Design review of the part built by this model. Coordinates are the model's own, in mm. A direction names the side the tool comes from. Give positions to 0.01 mm unless a question says otherwise; leave off trailing zeros. Order: outer loops, then holes, each group sorted by start corner. A loop starts at its lowest first (then second) coordinate and runs counter-clockwise, first axis right, second up. Notation, with made-up numbers: (-21.5, -5) -> (26.5, -5) arc R33 cw to (26.5, 33) -> close; hole circle Ø1 at (-14, 10). An arc over 180 degrees is marked (long way). Answer in a Markdown table with one row per item. Add a question column.
```python
from build123d import *

# Parameters (mm, degrees)
F0_W      = 10
F0_H      = 104
F1_DEPTH  = 10
F2_W      = 10
F2_H      = 2
F3_DEPTH  = 15
F4_W      = 10
F4_H      = 2
F5_DEPTH  = 30
F7_DEPTH  = 10.001
F8_R      = 0.99999
F9_W      = 3
F9_H      = 15
F10_DEPTH = 7


# Not quite as in the source:
# - a fillet or chamfer is up to 0.001 mm smaller than in the source, because OpenCascade refuses the exact size


with BuildPart() as f1:
    # F0 (on Top) → F1 (new body)
    with BuildSketch(Plane.XY):
        Rectangle(F0_W, F0_H)
    extrude(amount=F1_DEPTH)

    # F2 (on face) → F3 (join)
    with BuildSketch(Plane.XY.offset(10)):
        with Locations((0, -51)):
            Rectangle(F2_W, F2_H)
    extrude(amount=F3_DEPTH)

    # F4 (on face) → F5 (join)
    with BuildSketch(Plane.XY.offset(10)):
        with Locations((0, 51)):
            Rectangle(F4_W, F4_H)
    extrude(amount=F5_DEPTH)

    # F6 (on face) → F7 (cut, through all)
    with BuildSketch(Plane.YZ.offset(5)):
        Polygon((47, 5), (-30.8395786217, 0), (47, 0), align=None)
    extrude(amount=-F7_DEPTH, mode=Mode.SUBTRACT)

    # F8 (radius 1 in the source; OpenCascade refuses exactly that, so slightly less here)
    f8_edges = [f1.edges().sort_by_distance(p)[0] for p in [
        (0, 50, 40),
        (0, 52, 40),
        (0, -52, 25),
        (0, -50, 25),
        (0, 50, 10),
        (0, -50, 10),
    ]]
    fillet(f8_edges, radius=F8_R)

    # F9 (on face) → F10 (cut)
    with BuildSketch(Plane(origin=(-5, 0, 0), x_dir=(0, -1, 0), z_dir=(-1, 0, 0))):
        with Locations((50.5, 17.5)):
            Rectangle(F9_W, F9_H)
    extrude(amount=-F10_DEPTH, mode=Mode.SUBTRACT)


solid = f1.part
```
1) For L1, parallel to Y at x = 4.5, z = 17.5; L2, parallel to Y at x = -1, z = 32; L3, parallel to Z at x = 3.5, y = -32, list the stretches that pass through material, from the lowest coordinate up.
2) Add section D-D, the plane z = 37. Write out the cut boundary in (x, y), and give its area (3 significant figures).
3) Add section A-A, the plane z = 18.5. Write out the cut boundary in (x, y), and give its area (3 significant figures).
4) Add section C-C, the plane y = -41.5. Write out the cut boundary in (x, z).
5) Mouldability with a two-part tool opening along Y and no side actions: class faces 1 (the face through (0, 50, 0)), 2 (the face through (1, -52, 9)), 3 (the face through (0, -1, 10)) as +Y half, -Y half, draft (parallel to the pull), parting line (faces both ways), or undercut.
6) Machinability: for faces 4 (the face through (0.07, 8.625, 2.535)), 5 (the face through (0, 50, 25)), 6 (the face through (5, -8, 8)), 7 (the face through (2, -51, 18)), 8 (the face through (0, 52, 19)), which of the approach directions +Z, -Z, +X, -X, +Y, -Y give a long, thin tool a straight path to every point of the face, cutting with its end or side? Answer none if there is none.
7) Clearance check with flat-ended pins moving along their axes: P1, Ø2.5, axis at y = -50.5, z = 18.5, coming from the -X side; P2, Ø2, axis at x = 4, y = -38.5, coming from the +Z side; P3, Ø6, axis at x = 2, z = 31, coming from the -Y side. State where each tip first meets the part, or that it passes through.
Verdict:
| question | item | result |
|---|---|---|
| 1 | L1 | y = -52 to -50, 50 to 52 |
| 1 | L2 | y = 50 to 52 |
| 1 | L3 | z = 0 to 10 |
| 2 | outline | (-5, 50) -> (5, 50) -> (5, 52) -> (-5, 52) -> close |
| 2 | area | 20.0 mm2 |
| 3 | outline | (-5, 50) -> (5, 50) -> (5, 52) -> (-5, 52) -> close; (2, -52) -> (5, -52) -> (5, -50) -> (2, -50) -> close |
| 3 | area | 26.0 mm2 |
| 4 | outline | (-5, 0) -> (5, 0) -> (5, 10) -> (-5, 10) -> close |
| 5 | face 1 | draft |
| 5 | face 2 | -Y half |
| 5 | face 3 | undercut |
| 6 | face 4 | -Z, +X, -X |
| 6 | face 5 | +Z, +X, -X |
| 6 | face 6 | +Z, -Z, +X, +Y, -Y |
| 6 | face 7 | +Z, -X, -Y |
| 6 | face 8 | +Z, -Z, +X, -X, +Y |
| 7 | P1 | stops at x = 2 |
| 7 | P2 | stops at z = 10 |
| 7 | P3 | stops at y = 50 |
